Geometry check sheet. Reference: the model listing, model coordinates, mm. A direction names the side the tool comes from. Give positions to 0.01 mm unless a question says otherwise; leave off trailing zeros. Write each loop counter-clockwise with the first axis right and the second up, starting at its lowest first coordinate (ties: lowest second). Pieces come first, ordered by that corner, then holes.
(1) Mould release check, pull along X, two halves, no side actions. Record for faces 1 (the flat face through (2, 4.8, 6)), 2 (the flat face through (-4.232, 2.366, -4.375)), 3 (the cylindrical face through (2.503, 2.366, -8.315)), 4 (the flat face through (-5.468, 2.366, 2.673)): +X half, -X half, draft (parallel to the pull), parting line (faces both ways), or undercut.
(2) Cross-section at A-A (y = 3.5). Count the separate pieces of the cut face and the enclosed holes in it, and give its area (3 significant figures).
(3) Cross-section at D-D (y = -0.5). Record the boundary of the cut face in (x, z).
(4) Depth check by flat-ended pin: P1, Ø5.5, axis at x = 0, z = 0, coming from the +Y side; P2, Ø1, axis at y = 2.5, z = -5.5, coming from the -X side; P3, Ø1, axis at x = -3, y = 3.5, coming from the -Z side; P4, Ø2, axis at x = 1.5, y = 0, coming from the -Z side. Enter the tip coordinate at first touch or a pass-through.
(5) Thickness scan on line 1 along X through (y, z) = (-1.3, 0); line 2 along Y through (x, z) = (-2.25, -7.5); line 3 along Z through (x, y) = (-3.5, 4.25). Record the ranges inside material, lowest first.
(6) Cross-section at C-C (x = -2). Record the boundary of the cut face in (y, z).
(7) Cross-section at B-B (z = 0). Record the boundary of the cut face in (x, y).
(8) Tool access check on faces 5 (the flat face through (2.853, 2.366, -5.376)), 6 (the flat face through (-5.628, 2.366, -2.422)), 7 (the flat face through (0.852, 2.366, 6.027)). Record the directions out of +Z, -Z, +X, -X, +Y, -Y that give a thin tool (end or side, any length) a straight path to the whole face; none if there is none.
```python
from build123d import *
from build123d.topology import SkipClean

# Parameters (mm, degrees)
BOSS_EXTRUDE1_DEPTH   = 4.8
BOSS_EXTRUDE1_2_DEPTH = 4.8
BOSS_EXTRUDE1_3_DEPTH = 4.8
BOSS_EXTRUDE1_4_DEPTH = 4.8
BOSS_EXTRUDE1_5_DEPTH = 4.8
BOSS_EXTRUDE2_START   = -1.7
SKETCH1_3_R           = 9.25
SKETCH1_3_R_2         = 4.65
BOSS_EXTRUDE2_DEPTH   = 1.7


with BuildPart() as part:
    # Sketch1 → Boss-Extrude1 (new body)
    with BuildSketch(Plane(origin=(0, 0, 0), x_dir=(1, 0, 0), z_dir=(0, 1, 0))):
        with BuildLine():
            ThreePointArc((-5.480218714, 5.235321016), (-7.1492914, 4.928406745), (-6.842377129, 3.259334059))
            Line((-6.842377129, 3.259334059), (-4.379874637, 1.561793252))
            ThreePointArc((-4.379874637, 1.561793252), (-3.828474728, 2.63918193), (-3.017716222, 3.537780209))
            Line((-3.017716222, 3.537780209), (-5.480218714, 5.235321016))
        make_face()
    extrude(amount=BOSS_EXTRUDE1_DEPTH)



with BuildPart() as body_2:
    # Sketch1 → Boss-Extrude1 2 (new body)
    with BuildSketch(Plane(origin=(0, 0, 0), x_dir=(1, 0, 0), z_dir=(0, 1, 0))):
        with BuildLine():
            ThreePointArc((-2.838809346, -3.682887658), (-3.693074925, -2.82554377), (-4.297154517, -1.77678447))
            Line((-4.297154517, -1.77678447), (-6.672566882, -3.594194554))
            ThreePointArc((-6.672566882, -3.594194554), (-6.89644589, -5.276418733), (-5.214221711, -5.500297741))
            Line((-5.214221711, -5.500297741), (-2.838809346, -3.682887658))
        make_face()
    extrude(amount=BOSS_EXTRUDE1_2_DEPTH)


with BuildPart() as body_3:
    # Sketch1 → Boss-Extrude1 3 (new body)
    with BuildSketch(Plane(origin=(0, 0, 0), x_dir=(1, 0, 0), z_dir=(0, 1, 0))):
        with BuildLine():
            Line((0.985400081, 7.51467697), (0.131897954, 4.648128971))
            ThreePointArc((0.131897954, 4.648128971), (1.326947418, 4.456647905), (2.432103324, 3.963252884))
            Line((2.432103324, 3.963252884), (3.285605451, 6.829800884))
            ThreePointArc((3.285605451, 6.829800884), (2.47794081, 8.322341612), (0.985400081, 7.51467697))
        make_face()
    extrude(amount=BOSS_EXTRUDE1_3_DEPTH)


with BuildPart() as body_4:
    # Sketch1 → Boss-Extrude1 4 (new body)
    with BuildSketch(Plane(origin=(0, 0, 0), x_dir=(1, 0, 0), z_dir=(0, 1, 0))):
        with BuildLine():
            ThreePointArc((2.625393974, -3.837943001), (1.546028901, -4.385464016), (0.361928675, -4.635893402))
            Line((0.361928675, -4.635893402), (1.356345588, -7.456655412))
            ThreePointArc((1.356345588, -7.456655412), (2.887053438, -8.189412861), (3.619810887, -6.658705012))
            Line((3.619810887, -6.658705012), (2.625393974, -3.837943001))
        make_face()
    extrude(amount=BOSS_EXTRUDE1_4_DEPTH)


with BuildPart() as body_5:
    # Sketch1 → Boss-Extrude1 5 (new body)
    with BuildSketch(Plane(origin=(0, 0, 0), x_dir=(1, 0, 0), z_dir=(0, 1, 0))):
        with BuildLine():
            Line((7.451387872, 1.384991723), (4.461392056, 1.310908436))
            ThreePointArc((4.461392056, 1.310908436), (4.648573334, 0.115177951), (4.52083874, -1.08835522))
            Line((4.52083874, -1.08835522), (7.510834557, -1.014271933))
            ThreePointArc((7.510834557, -1.014271933), (8.680743042, 0.215083237), (7.451387872, 1.384991723))
        make_face()
    extrude(amount=BOSS_EXTRUDE1_5_DEPTH)


with BuildPart() as part_1:
    with SkipClean():  # the faces are left unmerged after this step: merging them gives an invalid solid
        add(part.part)

        add(body_2.part)  # Boss-Extrude2 merges body 2

        add(body_3.part)  # Boss-Extrude2 merges body 3

        add(body_4.part)  # Boss-Extrude2 merges body 4

        add(body_5.part)  # Boss-Extrude2 merges body 5
        # Sketch1_3 → Boss-Extrude2 (add)
        with BuildSketch(Plane(origin=(0, 0, 0), x_dir=(1, 0, 0), z_dir=(0, 1, 0)).offset(BOSS_EXTRUDE2_START)):
            with Locations(Location((0, 0, 0), (0, 0, 270))):
                Circle(SKETCH1_3_R)
            with Locations(Location((0, 0, 0), (0, 0, 88.374578531))):
                Circle(SKETCH1_3_R_2, mode=Mode.SUBTRACT)
        extrude(amount=BOSS_EXTRUDE2_DEPTH)


solid = part_1.part
```
Reply:
1. face 1: draft
1. face 2: undercut
1. face 3: parting line
1. face 4: -X half
2. separate pieces: 5
2. enclosed holes: 0
2. area: 45.9 mm2
3. outline: circle Ø18.5 at (0, 0); hole circle Ø9.3 at (0, 0)
4. P1: passes through
4. P2: stops at x = -7.1
4. P3: stops at z = -3.87
4. P4: stops at z = -9.24
5. line 1: x = -9.25 to -4.65, 4.65 to 9.25
5. line 2: y = -1.7 to 0
5. line 3: z = -3.87 to -3.06, 3.06 to 4.19
6. outline: (-1.7, -9.03) - (0, -9.03) - (0, -4.2) - (-1.7, -4.2) - close; (-1.7, 4.2) - (0, 4.2) - (0, 9.03) - (-1.7, 9.03) - close
7. outline: (-9.25, -1.7) - (-4.65, -1.7) - (-4.65, 0) - (-9.25, 0) - close; (4.65, -1.7) - (9.25, -1.7) - (9.25, 0) - (8.67, 0) - (8.67, 4.8) - (4.65, 4.8) - close
8. face 5: +X, +Y
8. face 6: -X, +Y
8. face 7: +Z, +Y
